Geometry: final body of the model. Coordinates: model frame, mm. A direction names the side the tool comes from. Round coordinates to 2 decimals unless told otherwise and drop trailing zeros. Order: outer loops, then holes, each group sorted by start corner. A loop starts at its lowest first (then second) coordinate and runs counter-clockwise, first axis right, second up. Notation, with made-up numbers: (-35, -11) -> (2, -11) arc R25 ccw to (2, 24) -> close; hole circle Ø1 at (25, 43.25). An arc over 180 degrees is marked (long way). Put each result on its own line as item: value.
```python
from build123d import *

# Parameters (mm, degrees)
CYLINDER005_R     = 2.5
CYLINDER005_DEPTH = 90
CYLINDER004_R     = 7
CYLINDER004_DEPTH = 150
CYLINDER003_R     = 11
CYLINDER003_DEPTH = 31
PAD010_DEPTH      = 7


with BuildPart() as vis_d:
    # Cylinder005 → Cylinder005 (new body)
    with BuildSketch(Plane(origin=(32.5, 0, -12), x_dir=(1, 0, 0), z_dir=(0, 0, 1))):
        Circle(CYLINDER005_R)
    extrude(amount=CYLINDER005_DEPTH)


with BuildPart() as vis:
    # Part__Mirroring003: instance of vis_d
    add(vis_d.part.mirror(Plane(origin=(0, 0, 0), x_dir=(0, -1, 0), z_dir=(1, 0, 0))))

    # Fusion005: union vis_d
    add(vis_d.part)


with BuildPart() as axe:
    # Cylinder004 → Cylinder004 (new body)
    with BuildSketch(Plane.XY.offset(-50)):
        Circle(CYLINDER004_R)
    extrude(amount=CYLINDER004_DEPTH)


with BuildPart() as clone_of_ball_slider:
    # Cylinder003 → Cylinder003 (new body)
    with BuildSketch(Plane.XY):
        Circle(CYLINDER003_R)
    extrude(amount=CYLINDER003_DEPTH)

    # Fusion003: union axe
    add(axe.part)


with BuildPart() as clone_of_ball_slider_1:
    # Clone017 placement: moved
    add(clone_of_ball_slider.part.moved(Location((-77, -3, 13))))


with BuildPart() as part_mirroring002:
    # Part__Mirroring002: instance of Clone of ball slider
    add(clone_of_ball_slider_1.part.mirror(Plane(origin=(0, 0, 0), x_dir=(0, -1, 0), z_dir=(1, 0, 0))))


with BuildPart() as vis_sliders:
    # Fusion004 base: copy of Clone of ball slider
    add(clone_of_ball_slider_1.part)

    # Fusion004: union Part__Mirroring002
    add(part_mirroring002.part)

    # Fusion006: union vis
    add(vis.part)


with BuildPart() as cut006006:
    # Sketch → Pad010 (new body)
    with BuildSketch(Plane.XY.offset(25)):
        with BuildLine():
            Line((96.936684, 16), (96.936684, -22))
            Line((96.936684, -22), (-96.936684, -22))
            Line((-96.936684, -22), (-96.936684, 16))
            Line((-96.936684, 16), (-31.668603, 16))
            ThreePointArc((-31.668603, 16), (-26.011749, 18.343146), (-23.668603, 24))
            Line((-23.668603, 24), (-23.668603, 42.983311))
            ThreePointArc((-18.668603, 47.983311), (-22.204137, 46.518845), (-23.668603, 42.983311))
            Line((-18.668603, 47.983311), (18.668603, 47.983311))
            ThreePointArc((23.668603, 42.983311), (22.204137, 46.518845), (18.668603, 47.983311))
            Line((23.668603, 42.983311), (23.668603, 24))
            ThreePointArc((23.668603, 24), (26.011749, 18.343146), (31.668603, 16))
            Line((31.668603, 16), (96.936684, 16))
        make_face()
    extrude(amount=PAD010_DEPTH)


with BuildPart() as cut006006_1:
    # Clone016 placement: moved
    add(cut006006.part.moved(Location((0, 0, -32))))

    # Cut006006: cut vis sliders
    add(vis_sliders.part, mode=Mode.SUBTRACT)


solid = cut006006_1.part
```
1. Cut plane D-D on x = 39.5. Return loops of the section in (y, z).
Ans:
outline: (-22, -7) -> (16, -7) -> (16, 0) -> (-22, 0) -> close
2. Contact query for flat-ended pins moving along their axis: P1, Ø2, axis at x = -80, z = -4.5, coming from the +Y side; P2, Ø4, axis at x = 32.5, y = 0, coming from the +Z side. Output: stop coordinate, or through.
Ans:
P1: y = 16
P2: through
3. Draft query along Y for faces 1 (the face through (1, -22, -4)), 2 (the face through (-34.81, -0.96, -3.55)), 3 (the face through (22.24, 46.48, -3.55)), 4 (the face through (34.81, -0.96, -3.55)). Return one class per face: +Y half, -Y half, draft (parallel to the pull), parting line (faces both ways), or undercut.
Ans:
face 1: -Y half
face 2: undercut
face 3: +Y half
face 4: undercut
4. Material intervals for probe 1 along X at (y, z) = (-5.5, -2.75); probe 2 along Y at (x, z) = (-77, -2); probe 3 along X at (y, z) = (2, -0.5), sorted ascending.
Ans:
probe 1: -96.94 to -83.54, -70.46 to 70.46, 83.54 to 96.94
probe 2: -22 to -10, 4 to 16
probe 3: -96.94 to -81.9, -72.1 to -34, -31 to 31, 34 to 72.1, 81.9 to 96.94
5. Cut plane B-B on z = -2. Return loops of the section in (x, y).
Ans:
outline: (-96.94, -22) -> (96.94, -22) -> (96.94, 16) -> (31.67, 16) arc R8 cw to (23.67, 24) -> (23.67, 42.98) arc R5 ccw to (18.67, 47.98) -> (-18.67, 47.98) arc R5 ccw to (-23.67, 42.98) -> (-23.67, 24) arc R8 cw to (-31.67, 16) -> (-96.94, 16) -> close; hole circle Ø14 at (-77, -3); hole circle Ø5 at (-32.5, 0); hole circle Ø5 at (32.5, 0); hole circle Ø14 at (77, -3)
6. Cut plane C-C on y = 0. Return loops of the section in (x, z).
Ans:
outline: (-96.94, -7) -> (-83.32, -7) -> (-83.32, 0) -> (-96.94, 0) -> close; (-70.68, -7) -> (-35, -7) -> (-35, 0) -> (-70.68, 0) -> close; (-30, -7) -> (30, -7) -> (30, 0) -> (-30, 0) -> close; (35, -7) -> (70.68, -7) -> (70.68, 0) -> (35, 0) -> close; (83.32, -7) -> (96.94, -7) -> (96.94, 0) -> (83.32, 0) -> close
7. Cut plane A-A on x = -77. Return loops of the section in (y, z).
Ans:
outline: (-22, -7) -> (-10, -7) -> (-10, 0) -> (-22, 0) -> close; (4, -7) -> (16, -7) -> (16, 0) -> (4, 0) -> close
8. Set-up query: faces 5 (the face through (-23.669, 33, -4)), 6 (the face through (82.16, 1.73, -3.55)), 7 (the face through (23.669, 34, -4)). Return all of +Z, -Z, +X, -X, +Y, -Y with unobstructed straight access to the full face (end or side cutting, diameter ignored); none if empty.
Ans:
face 5: +Z, -Z, -X, +Y
face 6: +Z, -Z
face 7: +Z, -Z, +X, +Y
